Design review of the part shown in the three views and the two pictorial views. Dimensions are in mm from the part's minimum x, y and z. A direction names the side the tool comes from. Give positions to 0.01 mm unless a question says otherwise; leave off trailing zeros. Loops run counter-clockwise (first coordinate to the right, second up) from the corner with the lowest first, then second, coordinate; pieces in that order, holes last. Notation, with made-up numbers: (85, 16) - (129, 16) arc R24 ccw to (129, 49) - close; hole circle Ø10 at (-15, 12.5). An arc over 180 degrees is marked (long way). Answer in a Markdown table with one row per item.
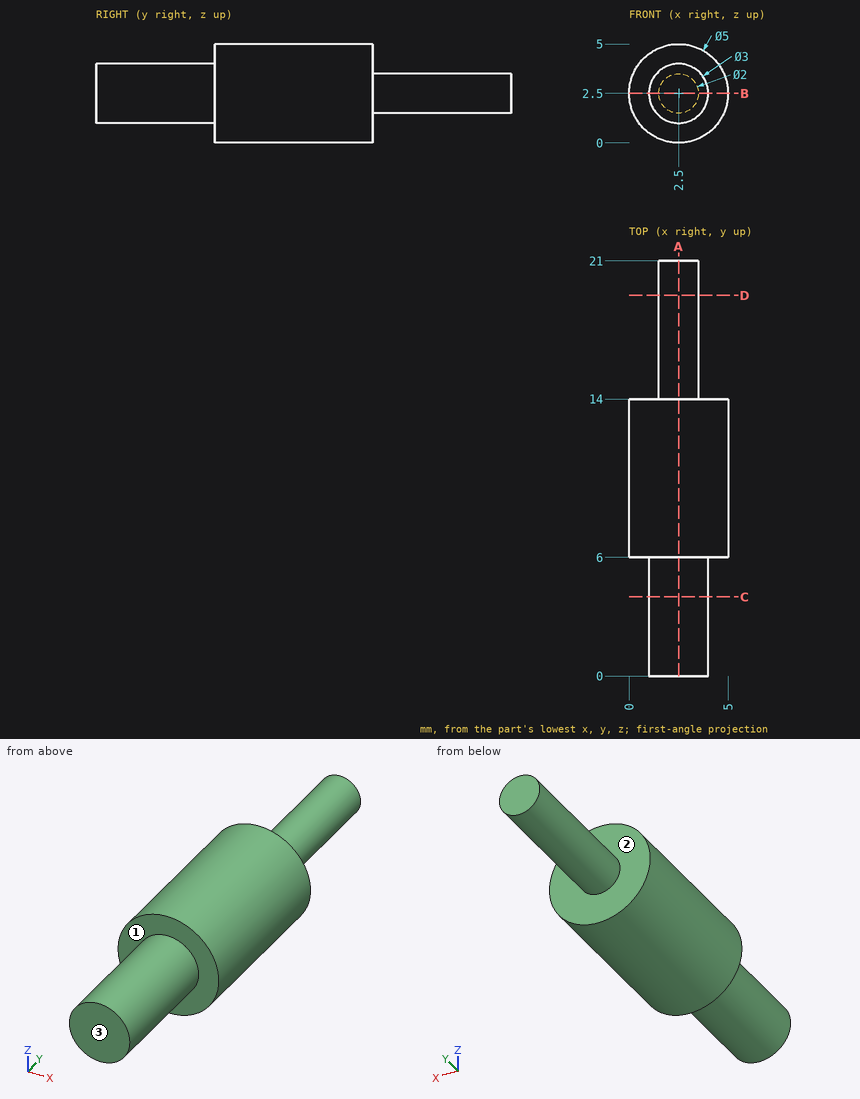
1. We need section C-C, the plane y = 4. Give the boundary of the cut face in (x, z), and give its area (3 significant figures).
Values:
| item | result |
|---|---|
| outline | circle Ø3 at (2.5, 2.5) |
| area | 7.07 mm^2 |
2. Wall thickness on line 1 (Y direction, x = 1.45, z = 0.8); line 2 (Y direction, x = 3.25, z = 3.5); line 3 (Z direction, x = 4.5, y = 11.5): over which ranges is each line inside the solid? List them lowest first. Write a range as [from, to].
Values:
| item | result |
|---|---|
| line 1 | y = [6, 14] |
| line 2 | y = [0, 14] |
| line 3 | z = [1, 4] |
3. We need section D-D, the plane y = 19.25. Give the boundary of the cut face in (x, z).
Values:
| item | result |
|---|---|
| outline | circle Ø2 at (2.5, 2.5) |
4. For the marked faces 1, 2 and 3, list the 3-axis set-ups (+Z, -Z, +X, -X, +Y, -Y) from which the entire face can be reached by the end or side of a thin tool; tool diameter is ignored.
Values:
| item | result |
|---|---|
| face 1 | -Y |
| face 2 | +Y |
| face 3 | +Z, -Z, +X, -X, -Y |
5. We need section A-A, the plane x = 2.5. Give the boundary of the cut face in (y, z), and give its area (3 significant figures).
Values:
| item | result |
|---|---|
| outline | (0, 1) - (6, 1) - (6, 0) - (14, 0) - (14, 1.5) - (21, 1.5) - (21, 3.5) - (14, 3.5) - (14, 5) - (6, 5) - (6, 4) - (0, 4) - close |
| area | 72.0 mm^2 |
6. Clearance check with flat-ended pins moving along their axes: pin 1 (1.5 mm diameter, centred on y = 18.5, z = 1.5, fed in from -X); pin 2 (2 mm diameter, centred on y = 11.5, z = 1, fed in from +X). State where each tip first meets the part, or that it passes through.
Values:
| item | result |
|---|---|
| pin 1 | stops at x = 1.53 |
| pin 2 | stops at x = 4.95 |
7. We need section B-B, the plane z = 2.5. Give the boundary of the cut face in (x, y), and give its area (3 significant figures).
Values:
| item | result |
|---|---|
| outline | (0, 6) - (1, 6) - (1, 0) - (4, 0) - (4, 6) - (5, 6) - (5, 14) - (3.5, 14) - (3.5, 21) - (1.5, 21) - (1.5, 14) - (0, 14) - close |
| area | 72.0 mm^2 |
